Read the model definition and answer for the solid it produces. Units are mm, in the model's axes. Face numbers are marked on the shaded views. A direction names the side the tool comes from. Give positions to 0.01 mm unless a question says otherwise; leave off trailing zeros. Use a Markdown table: item, result.
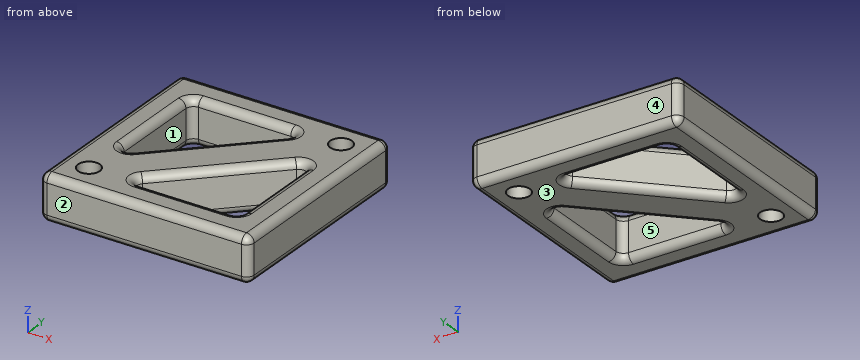
from build123d import *

# Parameters (mm, degrees)
SKETCH1_W           = 44.05525725
SKETCH1_H           = 44.45
BOSS_EXTRUDE1_DEPTH = 9.525
SKETCH2_R           = 2.286
CUT_EXTRUDE1_DEPTH  = 64.303979467
CUT_EXTRUDE2_DEPTH  = 64.303979467
FILLET1_R           = 1.5875


with BuildPart() as part:
    # Sketch1 → Boss-Extrude1 (new body)
    with BuildSketch(Plane.XY):
        with Locations((22.027628625, 22.225)):
            Rectangle(SKETCH1_W, SKETCH1_H)
    extrude(amount=BOSS_EXTRUDE1_DEPTH)

    # Sketch2 → Cut-Extrude1 (cut, through all)
    with BuildSketch(Plane(origin=(0, 0, 0), x_dir=(-1, 0, 0), z_dir=(0, 0, -1))):
        with Locations((-37.902628625, 38.1)):
            Circle(SKETCH2_R)
        with Locations((-6.152628625, 6.35)):
            Circle(SKETCH2_R)
    extrude(amount=-CUT_EXTRUDE1_DEPTH, mode=Mode.SUBTRACT)

    # Sketch3 → Cut-Extrude2 (cut, through all)
    with BuildSketch(Plane(origin=(0, 0, 0), x_dir=(-1, 0, 0), z_dir=(0, 0, -1))):
        Polygon((-31.167436534, 38.1), (-6.35, 38.1), (-6.35, 13.282563466), align=None)
        Polygon((-37.70525725, 31.167436534), (-12.887820716, 6.35), (-37.70525725, 6.35), align=None)
    extrude(amount=-CUT_EXTRUDE2_DEPTH, mode=Mode.SUBTRACT)

    # Fillet1
    fillet1_edges = [part.edges().sort_by_distance(p)[0] for p in [
        (44.05525725, 22.225, 9.525),
        (22.027628625, 44.45, 9.525),
        (37.70525725, 18.758718267, 9.525),
        (37.70525725, 6.35, 4.7625),
        (25.296538983, 18.758718267, 9.525),
        (37.70525725, 31.167436534, 4.7625),
        (25.296538983, 6.35, 9.525),
        (12.887820716, 6.35, 4.7625),
        (37.70525725, 18.758718267, 0),
        (25.296538983, 6.35, 0),
        (25.296538983, 18.758718267, 0),
        (18.758718267, 25.691281733, 9.525),
        (6.35, 13.282563466, 4.7625),
        (18.758718267, 38.1, 9.525),
        (31.167436534, 38.1, 4.7625),
        (6.35, 25.691281733, 9.525),
        (6.35, 38.1, 4.7625),
        (18.758718267, 25.691281733, 0),
        (6.35, 25.691281733, 0),
        (18.758718267, 38.1, 0),
        (0, 22.225, 9.525),
        (22.027628625, 44.45, 0),
        (44.05525725, 22.225, 0),
        (22.027628625, 0, 0),
        (0, 22.225, 0),
        (0, 44.45, 4.7625),
        (44.05525725, 44.45, 4.7625),
        (44.05525725, 0, 4.7625),
        (0, 0, 4.7625),
        (22.027628625, 0, 9.525),
    ]]
    fillet(fillet1_edges, radius=FILLET1_R)


solid = part.part
Item 1: For a pull along Y with two mould halves and no side action, classify the marked faces 3, 4 and 5 as +Y half, -Y half, draft (parallel to the pull), parting line (faces both ways), or undercut.
Return value:
| item | result |
|---|---|
| face 3 | draft |
| face 4 | +Y half |
| face 5 | undercut |
Item 2: Straight lines are drawn through the part: line 1 along Y through (x, z) = (38, 3.75); line 2 along X through (y, z) = (16, 9); line 3 along Y through (x, z) = (19.5, 2). For each, find the intervals that lie inside material, in ascending order. Write a range as [from, to].
Return value:
| item | result |
|---|---|
| line 1 | [0, 35.82], [40.38, 44.45] |
| line 2 | [0.41, 6.28], [9.64, 21.96], [38.11, 43.65] |
| line 3 | [0, 6.35], [12.96, 26.43], [38.1, 44.45] |
Item 3: This flat-tipped pin is pushed along its axis until it touches: P1, Ø2.5, axis at x = 6.15, y = 6.35, coming from the +Z side. Where does it stop, or does it pass through?
Return value:
| item | result |
|---|---|
| P1 | through |
Item 4: A tool of negligible diameter and unlimited length cuts with its end or side. For the marked faces 1 and 2, from which of +Z, -Z, +X, -X, +Y, -Y can it reach the whole face along a straight path? Write none if from no direction.
Return value:
| item | result |
|---|---|
| face 1 | +Z, -Z |
| face 2 | +Z, -Z, +X, -X, -Y |
Item 5: A cutting plane is placed at A-A (z = 2.5). Count the separate pieces of the cut face and the enclosed holes in it, then the cut area to 3 significant figures.
Return value:
| item | result |
|---|---|
| separate pieces | 1 |
| enclosed holes | 4 |
| area | 1,320 mm^2 |
